Print and shaded views of the part. All mm, measured from the part's lowest x, y and z. Round coordinates to 2 decimals unless told otherwise and drop trailing zeros. Order: outer loops, then holes, each group sorted by start corner. A loop starts at its lowest first (then second) coordinate and runs counter-clockwise, first axis right, second up. Notation, with made-up numbers: M 51,19 L 76,19 A20 cw 76,50 Z; hole C 0,-36 d11. An arc over 180 degrees is marked long. Write each question's results on one line, items separated by ' | '. Start each with the question number.
1. Band-saw the part on A-A, the plane x = 16. List the corners of the cut face in (y, z).
2. Band-saw the part on D-D, the plane x = 2.75. List the corners of the cut face in (y, z).
3. Drop flat-ended pins along their axis: pin 1 Ø1.2 at (y, z) = (35.5, 1) entering from +X; pin 2 Ø1.2 at (y, z) = (61, 1) entering from +X. Give the stop position or say it passes through.
4. Band-saw the part on B-B, the plane z = 1.75. List the corners of the cut face in (x, y), then the cut area to 3 significant figures.
5. Probe L1, parallel to Y at x = 19, z = 2.05; L2, parallel to X at y = 97, z = 2; L3, parallel to Y at x = 5.25, z = 2.45. List the from-to ranges inside material, lowest first. Write a range as [from, to].
6. Band-saw the part on C-C, the plane y = 14. List the corners of the cut face in (x, z), then the cut area to 3 significant figures.
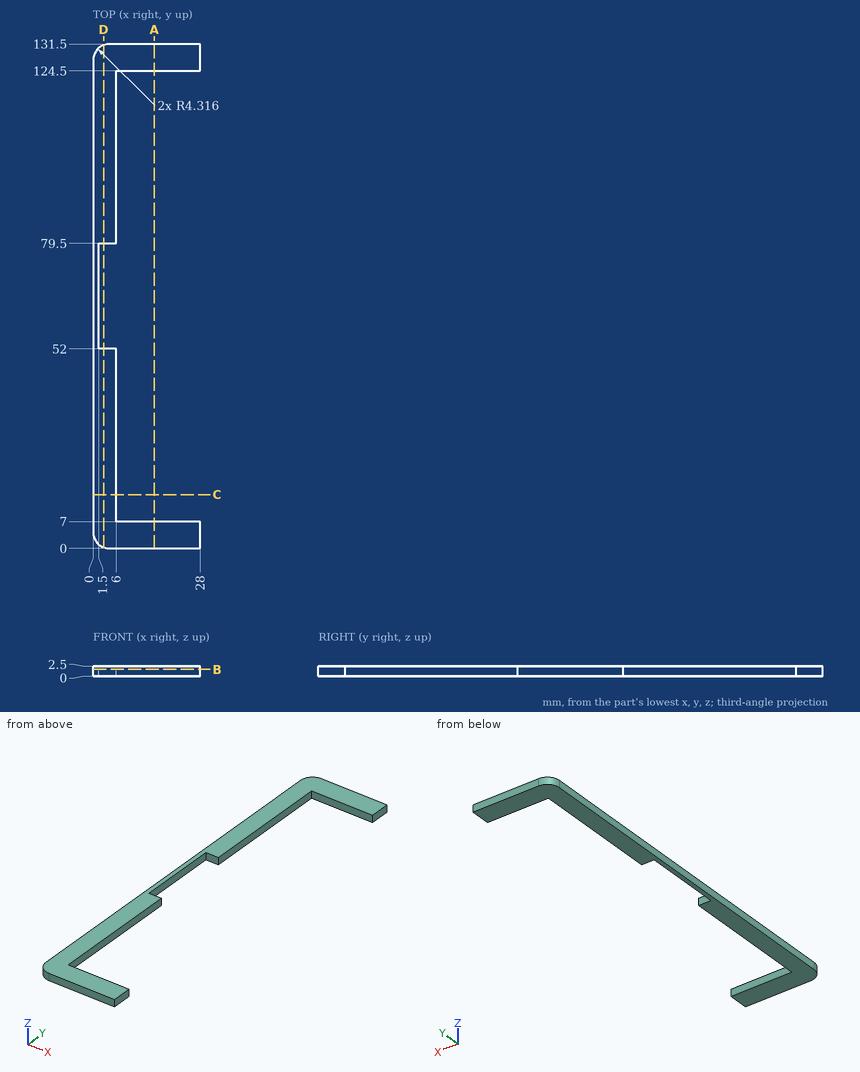
Solution:
1) outline: M 0,0 L 7,0 L 7,2.5 L 0,2.5 Z; M 124.5,0 L 131.5,0 L 131.5,2.5 L 124.5,2.5 Z
2) outline: M 0.29,0 L 52,0 L 52,2.5 L 0.29,2.5 Z; M 79.5,0 L 131.21,0 L 131.21,2.5 L 79.5,2.5 Z
3) pin 1: x = 6 | pin 2: x = 1.5
4) outline: M 0,4.32 A4.32 ccw 4.32,0 L 28,0 L 28,7 L 6,7 L 6,52 L 1.5,52 L 1.5,79.5 L 6,79.5 L 6,124.5 L 28,124.5 L 28,131.5 L 4.32,131.5 A4.32 ccw 0,127.18 Z | area: 965 mm^2
5) L1: [0, 7], [124.5, 131.5] | L2: [0, 6] | L3: [0, 52], [79.5, 131.5]
6) outline: M 0,0 L 6,0 L 6,2.5 L 0,2.5 Z | area: 15.0 mm^2
